Could you check a few things on this model? Use its own coordinates, in mm. Face numbers are marked on the shaded views. A direction names the side the tool comes from. Coordinates: 2 decimals unless noted, no trailing zeros. Loops run counter-clockwise (first coordinate to the right, second up) from the corner with the lowest first, then second, coordinate; pieces in that order, holes last. Notation, with made-up numbers: M 81.25,-20 L 117.25,-20 A15 cw 117.25,4 Z; hole C 2,71.25 d10. An arc over 180 degrees is marked long. Write each question's results on one line, items separated by ' | '.
```python
from build123d import *

# Parameters (mm, degrees)
SKETCH1_R           = 16.5
BOSS_EXTRUDE1_DEPTH = 82
SKETCH2_R           = 11
CUT_EXTRUDE1_DEPTH  = 276.268959383
SKETCH5_W           = 65
SKETCH5_H           = 35
CUT_EXTRUDE2_DEPTH  = 282.890049487
CUT_EXTRUDE3_DEPTH  = 40
SKETCH9_R           = 11
CUT_EXTRUDE4_DEPTH  = 22
SKETCH10_R          = 16.5
CUT_EXTRUDE5_DEPTH  = 57


with BuildPart() as part:
    # Sketch1 → Boss-Extrude1 (new body)
    with BuildSketch(Plane(origin=(0, 0, 0), x_dir=(1, 0, 0), z_dir=(0, 1, 0))):
        with BuildLine():
            Line((212.202700724, 100), (157.202700724, 100))
            ThreePointArc((157.202700724, 100), (151.120923095, 80.283600356), (134.9891913, 67.419244043))
            ThreePointArc((134.9891913, 67.419244043), (109.260251558, 61.670356138), (83, 64))
            Line((83, 64), (31.098692591, 64))
            Line((31.098692591, 64), (0, 35))
            Line((0, 35), (0, 0))
            Line((0, 0), (75.238209296, 0))
            ThreePointArc((75.238209296, 0), (96.859957606, -4.428268766), (115, -17))
            Line((115, -17), (157, -17))
            Line((157, -17), (176.293691384, 13.876360515))
            ThreePointArc((176.293691384, 13.876360515), (193.729138228, 30.421981775), (217, 36.440235832))
            Line((217, 36.440235832), (243, 36.440235832))
            Line((243, 36.440235832), (243, 80))
            Line((243, 80), (212.202700724, 100))
        make_face()
        with Locations(Location((135, 43, 0), (0, 0, 270))):
            Circle(SKETCH1_R, mode=Mode.SUBTRACT)
    extrude(amount=BOSS_EXTRUDE1_DEPTH)

    # Sketch2 → Cut-Extrude1 (cut, through all)
    with BuildSketch(Plane(origin=(0, 82, 0), x_dir=(1, 0, 0), z_dir=(0, 1, 0))):
        with Locations(Location((30, 35, 0), (0, 0, 270))):
            Circle(SKETCH2_R)
    extrude(amount=-CUT_EXTRUDE1_DEPTH, mode=Mode.SUBTRACT)

    # Sketch5 → Cut-Extrude2 (cut, through all)
    with BuildSketch(Plane(origin=(0, 0, -100), x_dir=(-1, 0, 0), z_dir=(0, 0, -1))):
        with Locations((-210.5, 64.5)):
            Rectangle(SKETCH5_W, SKETCH5_H)
    extrude(amount=-CUT_EXTRUDE2_DEPTH, mode=Mode.SUBTRACT)

    # Sketch6 → Cut-Extrude3 (cut)
    with BuildSketch(Plane(origin=(0, 15, 0), x_dir=(-1, 0, 0), z_dir=(0, -1, 0))):
        with BuildLine():
            Line((0, 12), (0, 35))
            Line((0, 35), (-31.098692591, 64))
            Line((-31.098692591, 64), (-74.689647512, 64))
            ThreePointArc((-74.689647512, 64), (-49.282519579, 20.85341744), (0, 12))
        make_face()
    extrude(amount=-CUT_EXTRUDE3_DEPTH, mode=Mode.SUBTRACT)

    # Sketch9 → Cut-Extrude4 (cut)
    with BuildSketch(Plane(origin=(0, 82, 0), x_dir=(1, 0, 0), z_dir=(0, 1, 0))):
        with BuildLine():
            Line((85, 2.172610945), (85, 60.459646479))
            ThreePointArc((85, 60.459646479), (83.816874247, 60.721767227), (82.637433549, 61))
            Line((82.637433549, 61), (32.280424018, 61))
            Line((32.280424018, 61), (3, 33.695562875))
            Line((3, 33.695562875), (3, 3))
            Line((3, 3), (75.238209296, 3))
            ThreePointArc((75.238209296, 3), (80.136605217, 2.792782572), (85, 2.172610945))
        make_face()
        with Locations(Location((30, 35, 0), (0, 0, 90))):
            Circle(SKETCH9_R, mode=Mode.SUBTRACT)
    extrude(amount=-CUT_EXTRUDE4_DEPTH, mode=Mode.SUBTRACT)

    # Sketch10 → Cut-Extrude5 (cut)
    with BuildSketch(Plane(origin=(0, 82, 0), x_dir=(1, 0, 0), z_dir=(0, 1, 0))):
        with BuildLine():
            ThreePointArc((136.085176207, 64.626607818), (110.849591358, 58.779397637), (85, 60.459646479))
            Line((85, 60.459646479), (85, 2.172610945))
            ThreePointArc((85, 2.172610945), (101.887734543, -3.484926438), (116.262592289, -14))
            Line((116.262592289, -14), (155.337072846, -14))
            Line((155.337072846, -14), (173.749547096, 15.466118308))
            ThreePointArc((173.749547096, 15.466118308), (174.364131851, 16.425638226), (175, 17.371188115))
            Line((175, 17.371188115), (175, 97))
            Line((175, 97), (160.084094573, 97))
            ThreePointArc((160.084094573, 97), (152.729470491, 77.370012647), (136.085176207, 64.626607818))
        make_face()
        with Locations(Location((135, 43, 0), (0, 0, 270))):
            Circle(SKETCH10_R, mode=Mode.SUBTRACT)
    extrude(amount=-CUT_EXTRUDE5_DEPTH, mode=Mode.SUBTRACT)


solid = part.part
```
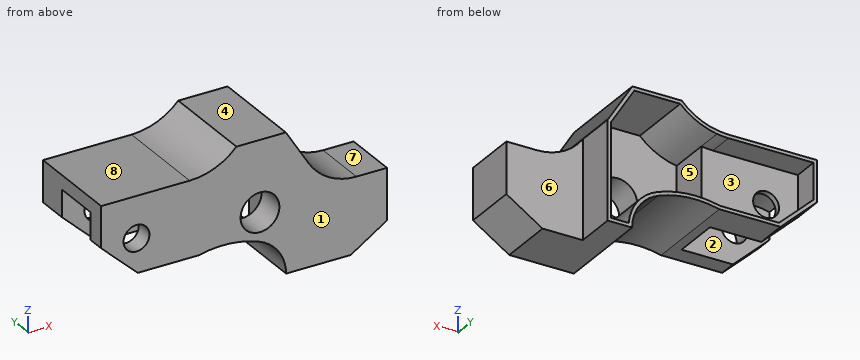
(1) Imagine slicing it at B-B, the plane z = -43. List the corners of the cut face in (x, y) for me, and give its area (3 significant figures).
Reported:
outline: M 8.58,0 L 22.45,0 L 22.45,15 L 8.58,15 Z; M 8.58,55 L 22.45,55 L 22.45,60 L 12.98,60 L 12.98,82 L 8.58,82 Z; M 37.55,0 L 118.5,0 L 118.5,25 L 85,25 L 85,60 L 37.55,60 L 37.55,55 L 68.53,55 L 68.53,15 L 37.55,15 Z; M 151.5,0 L 243,0 L 243,47 L 178,47 L 178,82 L 175,82 L 175,25 L 151.5,25 Z | area: 6,710 mm2
(2) Imagine slicing it at A-A, the plane y = 12. List the corners of the cut face in (x, z) for me, and give its area (3 significant figures).
Reported:
outline: M 0,-35 L 31.1,-64 L 83,-64 A85.85 cw 134.99,-67.42 A35 cw 157.2,-100 L 212.2,-100 L 243,-80 L 243,-36.44 L 217,-36.44 A48 cw 176.29,-13.88 L 157,17 L 115,17 A55 cw 75.24,0 L 0,0 Z; hole C 30,-35 d22; hole C 135,-43 d33 | area: 15,700 mm2
(3) Imagine slicing it at D-D, the plane z = -89. List the corners of the cut face in (x, y) for me.
Reported:
outline: M 155.43,0 L 229.14,0 L 229.14,47 L 178,47 L 178,82 L 175,82 L 175,25 L 158.58,25 L 158.58,82 L 155.43,82 Z
(4) Please list where these lines run through material, in increasing order: probe 1 along X at (y, z) = (58, -35); probe 2 along X at (y, z) = (9.5, -30); probe 3 along Z at (x, y) = (30, 58.1). Write a range as from..to.
Reported:
probe 1: x = 0..19, 41..85, 175..178 | probe 2: x = 0..20.2, 39.8..124.84, 145.16..192.98 | probe 3: z = -62.98..-46, -24..0
(5) If we mould it in two halves opening along Y, with no side actions, what happens to the marked faces 1, 2, 3 and 4? For each: released by +Y, released by -Y, zero draft, split by the parting line, or undercut.
Reported:
face 1: released by -Y | face 2: undercut | face 3: released by +Y | face 4: zero draft
(6) Will these pins go through, and if not, where does the flat tip stop? P1, Ø19.5, axis at x = 215.5, z = -51.5, coming from the +Y side; P2, Ø24, axis at y = 72.5, z = -18.5, coming from the +X side; P3, Ø6, axis at x = 137, y = 51.5, coming from the -Z side; P4, Ø20, axis at x = 30, z = -35, coming from the +Y side.
Reported:
P1: stops at y = 47 | P2: stops at x = 178 | P3: stops at z = -69.86 | P4: passes through
(7) Imagine slicing it at C-C, the plane y = 67.5. List the corners of the cut face in (x, z) for me.
Reported:
outline: M 0,-35 L 31.1,-64 L 83,-64 A85.85 cw 134.99,-67.42 A35 cw 157.2,-100 L 178,-100 L 178,-16.42 A48 cw 176.29,-13.88 L 157,17 L 115,17 A55 cw 75.24,0 L 0,0 Z; hole M 3,-33.7 L 32.28,-61 L 82.64,-61 A88.85 cw 85,-60.46 A88.85 cw 136.09,-64.63 A38 cw 160.08,-97 L 175,-97 L 175,-17.37 A51 cw 173.75,-15.47 L 155.34,14 L 116.26,14 A58 cw 75.24,-3 L 3,-3 Z
(8) Which directions (+Z, -Z, +X, -X, +Y, -Y) give clear straight access to the entire face, cutting with the end or side of a thin tool? Please do the marked faces 5, 6, 7 and 8.
Reported:
face 5: +Y | face 6: +Z, -Z, +X, +Y | face 7: +Z, +X, +Y, -Y | face 8: +Z, -X, +Y, -Y
